```python
from build123d import *

# Parameters (mm, degrees)
F0_W     = 20
F0_H     = 30
F0_R     = 2.5
F1_DEPTH = 13
F2_W     = 36
F2_H     = 17
F3_DEPTH = 3
F4_D     = 5.4
F5_DEPTH = 25
F6_R     = 2
F7_R     = 3.99999
F8_SIZE2 = 9
F8_SIZE  = 3
F9_SIZE  = 1


# Not quite as in the source:
# - a fillet or chamfer is up to 0.001 mm smaller than in the source, because OpenCascade refuses the exact size


with BuildPart() as f1:
    # F0 (on Top) → F1 (new body)
    with BuildSketch(Plane.XY):
        Polygon((-18, 20), (-18, 0), (18, 0), (18, 20), (10, 20), (-10, 20), align=None)
        with Locations((0, 35)):
            Rectangle(F0_W, F0_H)
        with Locations((0, 40)):
            Circle(F0_R, mode=Mode.SUBTRACT)
        with Locations((0, 40)):
            Circle(F0_R)
    extrude(amount=F1_DEPTH)

    # F2 (on face) → F3 (cut)
    with BuildSketch(Plane.XY.offset(13)):
        with Locations((0, 8.5)):
            Rectangle(F2_W, F2_H)
    extrude(amount=-F3_DEPTH, mode=Mode.SUBTRACT)

    # F4 (through all)
    with Locations(Plane(origin=(0, 0, 0), x_dir=(1, 0, 0), z_dir=(0, 0, -1))):
        with Locations((0, -21)):
            Hole(F4_D / 2)

    # F0 (on Top) → F5 (join)
    with BuildSketch(Plane.XY):
        with Locations((0, 40)):
            Circle(F0_R)
    extrude(amount=F5_DEPTH)

    # F6
    f6_edges = [f1.edges().sort_by_distance(p)[0] for p in [
        (-2.5, 40, 25),
    ]]
    fillet(f6_edges, radius=F6_R)

    # F7 (radius 4 in the source; OpenCascade refuses exactly that, so slightly less here)
    f7_edges = [f1.edges().sort_by_distance(p)[0] for p in [
        (-18, 20, 6.5),
        (18, 20, 6.5),
        (-10, 20, 6.5),
        (10, 20, 6.5),
    ]]
    fillet(f7_edges, radius=F7_R)

    # F8
    f8_edges = [f1.edges().sort_by_distance(p)[0] for p in [
        (0, 50, 0),
        (0, 0, 0),
    ]]
    f8_side = f1.faces().sort_by_distance((-17.383883, 8.000005, 0))[0]
    chamfer(f8_edges, length=F8_SIZE, length2=F8_SIZE2, reference=f8_side)

    # F9
    f9_edges = [f1.edges().sort_by_distance(p)[0] for p in [
        (16.82843, 18.82843, 0),
        (11.17157, 21.17157, 0),
        (-11.17157, 21.17157, 0),
        (-16.82843, 18.82843, 0),
        (18, 1.5, 4.5),
        (-18, 1.5, 4.5),
        (-10, 50, 11),
        (-10, 48.5, 4.5),
        (10, 50, 11),
        (10, 48.5, 4.5),
    ]]
    chamfer(f9_edges, length=F9_SIZE)


solid = f1.part
```
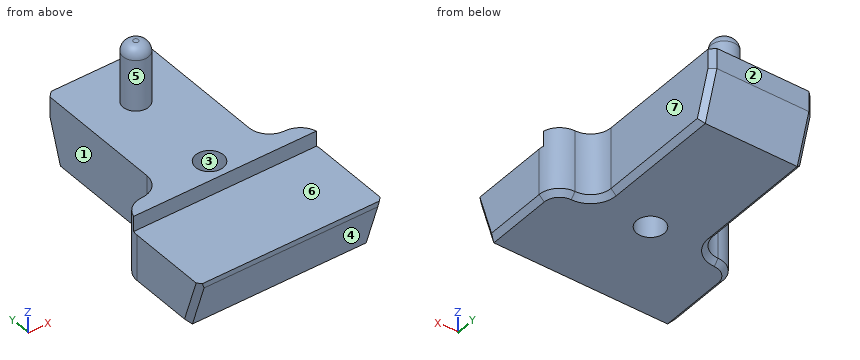
The listing builds one solid part. Answer for the finished solid, in the listing's coordinates (mm). Face numbers are marked on the shaded views. A direction names the side the tool comes from. Round coordinates to 2 decimals unless told otherwise and drop trailing zeros. Order: outer loops, then holes, each group sorted by start corner. A loop starts at its lowest first (then second) coordinate and runs counter-clockwise, first axis right, second up. Notation, with made-up numbers: (52, -27) - (56, -27) arc R17 cw to (56, 6) - close; hole circle Ø3 at (48, 10.5). An arc over 180 degrees is marked (long way). Put each result on its own line as item: value. Start each with the question number.
(1) Find section D-D (z = 15.5). Give the vertices of the cut face in (x, y), plus the area to 3 significant figures.
(2) Determine the mould class of the marked faces 1, 2 and 3 for opening direction Y: released by +Y, released by -Y, zero draft, split by the parting line, or undercut.
(3) For the marked faces 4, 5, 6 and 7, determine the directions among +Z, -Z, +X, -X, +Y, -Y from which every point of the face is accessible in a straight line to the end or side of a thin tool.
(4) Straight lines are drawn through the part: probe 1 along Y at (x, z) = (0, 6); probe 2 along Y at (x, z) = (0, 10.25); probe 3 along Z at (x, y) = (-14, 11). For each, find the intervals that lie inside material, in ascending order. Write a range as from..to.
(5) Find section C-C (y = 28.5). Give the vertices of the cut face in (x, z), plus the area to 3 significant figures.
(6) Find section A-A (x = -5.5). Give the vertices of the cut face in (y, z).
(7) Given P1, Ø9.5, axis at y = 36, z = 8, coming from the -X side; P2, Ø6, axis at y = 39, z = 5.5, coming from the +X side; P3, Ø0.9, axis at x = -5.5, z = 12, coming from the -Y side, each flat-ended and moving along its own axis, determine where each tip first touches the part or whether it passes through.
Reply:
1. outline: circle Ø5 at (0, 40)
1. area: 19.6 mm^2
2. face 1: zero draft
2. face 2: released by +Y
2. face 3: undercut
3. face 4: -Z, +X, -X, -Y
3. face 5: +Z
3. face 6: +Z, +X, -X, -Y
3. face 7: +Z, -Z, +X, +Y
4. probe 1: 1..18.3, 23.7..49
4. probe 2: 17..18.3, 23.7..50
4. probe 3: 0..10
5. outline: (-10, 1) - (-9, 0) - (9, 0) - (10, 1) - (10, 13) - (-10, 13) - close
5. area: 259 mm^2
6. outline: (0, 9) - (3, 0) - (47, 0) - (50, 9) - (50, 13) - (17, 13) - (17, 10) - (0, 10) - close
7. P1: x = -10
7. P2: x = 10
7. P3: y = 17
